```python
from build123d import *

# Parameters (mm, degrees)
SKETCH3_R               = 22.225
SKETCH3_R_2             = 21.336
BOSS_EXTRUDE1_DEPTH     = 400.05
CUT_EXTRUDE1_DEPTH      = 402.282822645
CUT_EXTRUDE1_DEPTH_BACK = 402.282822645
SKETCH4_R               = 2.5527
CIRPATTERN1_COUNT       = 3


# Read off the part's stored shape, not the designer's step: CSK for M3 SFHCS1
with BuildPart() as part:
    # Sketch3 → Boss-Extrude1 (new, symmetric)
    with BuildSketch(Plane(origin=(0, 0, 0), x_dir=(0, 0, -1), z_dir=(1, 0, 0))):
        with Locations(Location((0, 0, 0), (0, 0, 180))):
            Circle(SKETCH3_R)
        with Locations(Location((0, 0, 0), (0, 0, 180))):
            Circle(SKETCH3_R_2, mode=Mode.SUBTRACT)
    extrude(amount=BOSS_EXTRUDE1_DEPTH, both=True)

    # Sketch4 → Cut-Extrude1 (cut, two sides: drawn at the far end of the back side and taken through both)
    with BuildSketch(Plane.XY.offset(-CUT_EXTRUDE1_DEPTH_BACK)):
        with Locations(Location((336.55, 0, 0), (0, 0, 180))):
            Circle(SKETCH4_R)
        with Locations(Location((387.35, 0, 0), (0, 0, 180))):
            Circle(SKETCH4_R)
    extrude(amount=CUT_EXTRUDE1_DEPTH + CUT_EXTRUDE1_DEPTH_BACK, mode=Mode.SUBTRACT)

    # CSK for M3 SFHCS1 outline → CSK for M3 SFHCS1 (revolve, cut)
    with BuildSketch(Plane(origin=(-392.1125, 0, 0), x_dir=(1, 0, 0), z_dir=(0, -1, 0))):
        Polygon((3.360105502, 22.225105502), (0, 22.225105502), (0, 21.206997784), (2.341997784, 21.206997784), align=None)
    csk_for_m3_sfhcs1 = revolve(axis=Axis((-392.1125, 0, 0), (0, 0, 1)), mode=Mode.SUBTRACT)

    # CirPattern1: CSK for M3 SFHCS1 ×3 about axis
    cirpattern1_axis = Axis((400.05, 0, 0), (-1, 0, 0))
    for i in range(1, CIRPATTERN1_COUNT):
        add(csk_for_m3_sfhcs1.rotate(cirpattern1_axis, i * 360 / CIRPATTERN1_COUNT), mode=Mode.SUBTRACT)


solid = part.part
```
The model under review builds one solid part; all positions refer to its coordinate system, in mm. Give positions to 0.01 mm unless a question says otherwise; leave off trailing zeros. Write each loop counter-clockwise with the first axis right and the second up, starting at its lowest first coordinate (ties: lowest second). Pieces come first, ordered by that corner, then holes. Notation, with made-up numbers: (24, 11.5) -> (71, 11.5) arc R27 ccw to (71, 37.5) -> close; hole circle Ø9 at (-29.5, 18.5). An arc over 180 degrees is marked (long way). Answer in a Markdown table with one row per item.
1) Add section A-A on z = 0. State the section outline as (x, y) points (3 decimals).
Worked answers:
| item | result |
|---|---|
| outline | (-400.05, -22.225) -> (400.05, -22.225) -> (400.05, -21.336) -> (-400.05, -21.336) -> close; (-400.05, 21.336) -> (400.05, 21.336) -> (400.05, 22.225) -> (-400.05, 22.225) -> close |
2) Add section B-B on y = 10. State the section outline as (x, z) points.
Worked answers:
| item | result |
|---|---|
| outline | (-400.05, -19.85) -> (400.05, -19.85) -> (400.05, -18.85) -> (-400.05, -18.85) -> close; (-400.05, 18.85) -> (400.05, 18.85) -> (400.05, 19.85) -> (-400.05, 19.85) -> close |
3) Clearance check with flat-ended pins moving along their axes: P1, Ø4.5, axis at x = 387.35, y = 0, coming from the +Z side; P2, Ø6, axis at x = 291.5, z = 12, coming from the -Y side; P3, Ø3, axis at x = 267, y = 9, coming from the +Z side; P4, Ø4, axis at x = -82, y = 16, coming from the +Z side. State where each tip first meets the part, or that it passes through.
Worked answers:
| item | result |
|---|---|
| P1 | through |
| P2 | y = -20.32 |
| P3 | z = 20.92 |
| P4 | z = 17.26 |
4) Add section C-C on x = -169. State the section outline as (y, z) points (3 decimals).
Worked answers:
| item | result |
|---|---|
| outline | circle Ø44.45 at (0, 0); hole circle Ø42.672 at (0, 0) |
5) For L1, parallel to Y at x = 346, z = 2; L2, parallel to Z at x = -184.5, y = 0.5; L3, parallel to Z at x = -76, y = 2.5, list the stretches that pass through material, from the lowest coordinate up. Write a range as [from, to].
Worked answers:
| item | result |
|---|---|
| L1 | [-22.13, -21.24], [21.24, 22.13] |
| L2 | [-22.22, -21.33], [21.33, 22.22] |
| L3 | [-22.08, -21.19], [21.19, 22.08] |
6) Mouldability with a two-part tool opening along Z and no side actions: class faces 1 (the flat face through (400.05, -20, -8)), 2 (the cylindrical face through (-5.601, 18.929, 9.845)), 3 (the cylindrical face through (5.6, -15, -16.4)) as +Z half, -Z half, draft (parallel to the pull), parting line (faces both ways), or undercut.
Worked answers:
| item | result |
|---|---|
| face 1 | draft |
| face 2 | undercut |
| face 3 | parting line |
